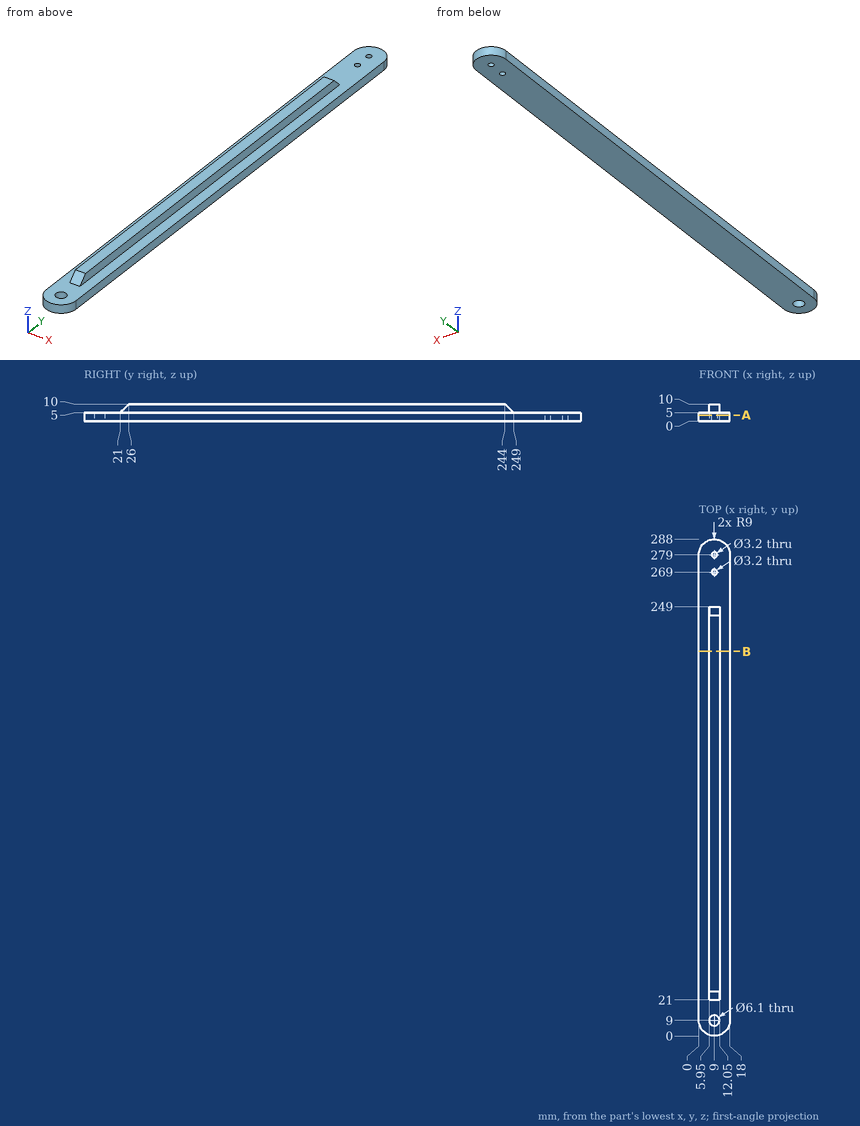
Drawing for the job (mm, zero at the part's lowest x, y, z). Coordinates: 2 decimals unless noted, no trailing zeros. Write each loop counter-clockwise with the first axis right and the second up, starting at its lowest first coordinate (ties: lowest second). Pieces come first, ordered by that corner, then holes. Notation, with made-up numbers: (71.25, 21) -> (111.25, 21) arc R18 ccw to (111.25, 47) -> close; hole circle Ø8 at (-33, 0.5). An arc over 180 degrees is marked (long way). One line per item, written item: value. Start each with the question number.
1) Slice it at B-B on y = 223. Write the cut outline in (x, z), then the cut area to 4 significant figures.
2) Probe probe 1 along Y at (x, z) = (9, 2.2); probe 2 along X at (y, z) = (269, 1.8); probe 3 along Y at (x, z) = (8.5, 1.5). List the from-to ranges inside material, lowest first.
3) Flat gauge pins, fed straight in: pin 1 Ø4 at (x, y) = (9, 269) entering from -Z; pin 2 Ø5 at (x, y) = (9, 9) entering from +Z; pin 3 Ø5.5 at (y, z) = (100, 8) entering from +X; pin 4 Ø1 at (y, z) = (86.5, 8.5) entering from -X. Where does each tip first touch, or does it go through?
4) Slice it at A-A on z = 3.5. Write the cut outline in (x, y), then the cut area to 3 significant figures.
Answers follow:
1. outline: (0, 0) -> (18, 0) -> (18, 5) -> (12.05, 5) -> (12.05, 10) -> (5.95, 10) -> (5.95, 5) -> (0, 5) -> close
1. area: 120.5 mm2
2. probe 1: 0 to 5.95, 12.05 to 267.4, 270.6 to 277.4, 280.6 to 288
2. probe 2: 0 to 7.4, 10.6 to 18
2. probe 3: 0.01 to 5.99, 12.01 to 267.48, 270.52 to 277.48, 280.52 to 287.99
3. pin 1: z = 0
3. pin 2: through
3. pin 3: x = 12.05
3. pin 4: x = 5.95
4. outline: (0, 9) arc R9 ccw to (18, 9) -> (18, 279) arc R9 ccw to (0, 279) -> close; hole circle Ø6.1 at (9, 9); hole circle Ø3.2 at (9, 269); hole circle Ø3.2 at (9, 279)
4. area: 5,070 mm2
